from build123d import *

# Parameters (mm, degrees)
SKETCH1_W                      = 80
SKETCH1_H                      = 360
BASE_FLANGE1_DEPTH             = 2
EDGE_FLANGE1_STRIP_W           = 12
EDGE_FLANGE1_STRIP_H           = 2
EDGE_FLANGE1_STRIP_CUT_DEPTH   = 360
EDGE_FLANGE1_STRIP_2_W         = 12
EDGE_FLANGE1_STRIP_2_H         = 2
EDGE_FLANGE1_STRIP_CUT_2_DEPTH = 360
EDGE_FLANGE1_DEPTH             = 360
EDGE_FLANGE1_BEND_DEPTH        = 360


# Sheet-metal steps are written as plain solids
with BuildPart() as part:
    # Sketch1 → Base-Flange1 (new body)
    with BuildSketch(Plane(origin=(0, 240, 0), x_dir=(1, 0, 0), z_dir=(0, 1, 0))):
        Rectangle(SKETCH1_W, SKETCH1_H)
    extrude(amount=BASE_FLANGE1_DEPTH)

    # Edge-Flange1 strip (across the edge) → Edge-Flange1 strip cut (cut)
    with BuildSketch(Plane(origin=(40, 240, -180), x_dir=(-1, 0, 0), z_dir=(0, 0, 1))):
        with Locations((-4, -1)):
            Rectangle(EDGE_FLANGE1_STRIP_W, EDGE_FLANGE1_STRIP_H)
    extrude(amount=EDGE_FLANGE1_STRIP_CUT_DEPTH, mode=Mode.SUBTRACT)

    # Edge-Flange1 strip 2 (across the edge) → Edge-Flange1 strip cut 2 (cut)
    with BuildSketch(Plane(origin=(-40, 240, 180), x_dir=(1, 0, 0), z_dir=(0, 0, -1))):
        with Locations((-4, -1)):
            Rectangle(EDGE_FLANGE1_STRIP_2_W, EDGE_FLANGE1_STRIP_2_H)
    extrude(amount=EDGE_FLANGE1_STRIP_CUT_2_DEPTH, mode=Mode.SUBTRACT)

    # Edge-Flange1 section (across the edge) → Edge-Flange1 (add)
    with BuildSketch(Plane(origin=(40, 240, -180), x_dir=(-1, 0, 0), z_dir=(0, 0, 1))):
        with BuildLine():
            Line((-2, 2), (-2, 36))
            Line((-2, 36), (0, 36))
            Line((0, 36), (0, 2))
            ThreePointArc((0, 2), (0.585786438, 0.585786438), (2, 0))
            Line((2, 0), (2, -2))
            ThreePointArc((2, -2), (-0.828427125, -0.828427125), (-2, 2))
        make_face()
    extrude(amount=EDGE_FLANGE1_DEPTH)

    # Edge-Flange1 section 2 (across the edge) → Edge-Flange1 bend (add)
    with BuildSketch(Plane(origin=(-40, 240, 180), x_dir=(1, 0, 0), z_dir=(0, 0, -1))):
        with BuildLine():
            Line((-2, 2), (-2, 36))
            Line((-2, 36), (0, 36))
            Line((0, 36), (0, 2))
            ThreePointArc((0, 2), (0.585786438, 0.585786438), (2, 0))
            Line((2, 0), (2, -2))
            ThreePointArc((2, -2), (-0.828427125, -0.828427125), (-2, 2))
        make_face()
    extrude(amount=EDGE_FLANGE1_BEND_DEPTH)


solid = part.part
Verification items for the finished model (mm, model axes). A direction names the side the tool comes from. Coordinates: 2 decimals unless noted, no trailing zeros. Write each loop counter-clockwise with the first axis right and the second up, starting at its lowest first coordinate (ties: lowest second). Pieces come first, ordered by that corner, then holes. Notation, with made-up numbers: M 75.25,39 L 129.25,39 A21 ccw 129.25,61 Z; hole C 87,56.25 d10. An arc over 180 degrees is marked long. Use a Markdown table: item, result.
Q1. Thickness scan on line 1 (X direction, y = 206.5, z = -23.5); line 2 (Y direction, x = 9, z = 104); line 3 (X direction, y = 239, z = -111). Record the ranges inside material, lowest first.
Reply:
| item | result |
|---|---|
| line 1 | x = -42 to -40, 40 to 42 |
| line 2 | y = 240 to 242 |
| line 3 | x = -41.87 to -39.73, 39.73 to 41.87 |
Q2. Sectioned sample at C-C, the plane x = -12. Record the boundary of the cut face in (y, z), plus the area to 3 significant figures.
Reply:
| item | result |
|---|---|
| outline | M 240,-180 L 242,-180 L 242,180 L 240,180 Z |
| area | 720 mm² |
Q3. Sectioned sample at A-A, the plane y = 220. Record the boundary of the cut face in (x, z).
Reply:
| item | result |
|---|---|
| outline | M -42,-180 L -40,-180 L -40,180 L -42,180 Z; M 40,-180 L 42,-180 L 42,180 L 40,180 Z |
Q4. Set-up check for faces 1 (the face through (-40, 221, 3)), 2 (the face through (0, 241, -180)): record each of +Z, -Z, +X, -X, +Y, -Y from which the full face is reachable in a straight line by a thin tool's end or side.
Reply:
| item | result |
|---|---|
| face 1 | +Z, -Z, -Y |
| face 2 | -Z, +X, -X, +Y, -Y |
Q5. Sectioned sample at B-B, the plane z = -129. Record the boundary of the cut face in (x, y), plus the area to 3 significant figures.
Reply:
| item | result |
|---|---|
| outline | M -42,204 L -40,204 L -40,238 A2 cw -38,240 L 38,240 A2 cw 40,238 L 40,204 L 42,204 L 42,238 A4 ccw 38,242 L -38,242 A4 ccw -42,238 Z |
| area | 307 mm² |
Q6. Go/stop test with a flat-tipped pin: P1, Ø8, axis at x = 10.5, z = -84.5, coming from the -Y side. Record where the tip stops, or that it passes through.
Reply:
| item | result |
|---|---|
| P1 | stops at y = 240 |
Q7. Draft check along X on faces 3 (the face through (-1, 242, -3)), 4 (the face through (-1, 240, -3)), 5 (the face through (42, 221, -3)), 6 (the face through (-42, 221, 3)). Enter one of: +X half, -X half, draft (parallel to the pull), parting line (faces both ways), or undercut.
Reply:
| item | result |
|---|---|
| face 3 | draft |
| face 4 | undercut |
| face 5 | +X half |
| face 6 | -X half |
